Design review of the part built by this model. Coordinates are the model's own, in mm. Face numbers are marked on the shaded views. A direction names the side the tool comes from. Give positions to 0.01 mm unless a question says otherwise; leave off trailing zeros. Order: outer loops, then holes, each group sorted by start corner. A loop starts at its lowest first (then second) coordinate and runs counter-clockwise, first axis right, second up. Notation, with made-up numbers: (-26.5, 32) -> (10.5, 32) arc R28 ccw to (10.5, 66) -> close; hole circle Ø8 at (-15.75, -23). An arc over 180 degrees is marked (long way). Return JSON: item names as keys, results as strings.
```python
from build123d import *

# Parameters (mm, degrees)
BOSS_EXTRUDE1_DEPTH = 32
FILLET1_R           = 10
SKETCH4_W           = 170.11041037
SKETCH4_H           = 258.008077424
CUT_EXTRUDE2_DEPTH  = 33
SKETCH6_R           = 1.2
CUT_EXTRUDE3_DEPTH  = 61.218304139
SKETCH7_R           = 1.2
CUT_EXTRUDE4_DEPTH  = 61.218304139


with BuildPart() as part:
    # Sketch1 → Boss-Extrude1 (new body)
    with BuildSketch(Plane(origin=(0, 0, 0), x_dir=(1, 0, 0), z_dir=(0, 1, 0))):
        Polygon((0, 0), (0, 30), (83, 115), (83, 107.843231513), (5, 27.963713441), (5, -27.963713441), (83, -107.843231513), (83, -115), (0, -30), align=None)
    extrude(amount=BOSS_EXTRUDE1_DEPTH)

    # Fillet1
    fillet1_edges = [part.edges().sort_by_distance(p)[0] for p in [
        (0, 16, 30),
        (0, 16, -30),
    ]]
    fillet(fillet1_edges, radius=FILLET1_R)

    # Sketch4 → Cut-Extrude2 (cut, through all)
    with BuildSketch(Plane(origin=(0, 32, 0), x_dir=(1, 0, 0), z_dir=(0, 1, 0))):
        with Locations((35.635219957, -4.046970822)):
            Rectangle(SKETCH4_W, SKETCH4_H)
        Polygon((14.577370106, -37.771863549), (11, -41.265060241), (0, -41.265060241), (0, 41.265060241), (11, 41.265060241), (14.577370106, 37.771863549), align=None, mode=Mode.SUBTRACT)
    extrude(amount=-CUT_EXTRUDE2_DEPTH, mode=Mode.SUBTRACT)

    # Sketch6 → Cut-Extrude3 (cut, through all)
    with BuildSketch(Plane(origin=(-14.995748902, 0, -14.642907751), x_dir=(-0.698639338, 0, 0.715474021), z_dir=(-0.715474021, 0, -0.698639338))):
        with Locations((-34.209111306, 26)):
            Circle(SKETCH6_R)
        with Locations((-34.209111306, 6)):
            Circle(SKETCH6_R)
    extrude(amount=-CUT_EXTRUDE3_DEPTH, mode=Mode.SUBTRACT)

    # Sketch7 → Cut-Extrude4 (cut, through all)
    with BuildSketch(Plane(origin=(-14.995748902, 0, 14.642907751), x_dir=(0.698639338, 0, 0.715474021), z_dir=(-0.715474021, 0, 0.698639338))):
        with Locations((34.209111306, 26)):
            Circle(SKETCH7_R)
        with Locations((34.209111306, 6)):
            Circle(SKETCH7_R)
    extrude(amount=-CUT_EXTRUDE4_DEPTH, mode=Mode.SUBTRACT)


solid = part.part
```
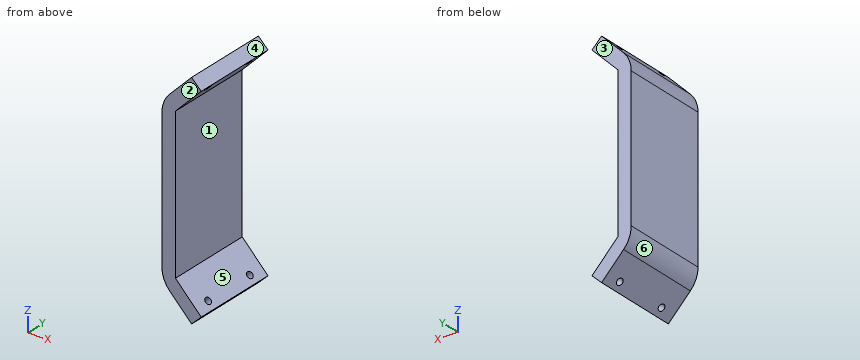
Item 1: Add section D-D (x = 1.25). Give the boundary of the cut face in (y, z), plus the area to 3 significant figures.
Result set:
{"outline": "(0, -30.77) -> (32, -30.77) -> (32, 30.77) -> (0, 30.77) -> close", "area": "1,970 mm^2"}
Item 2: For pin 1 (2 mm diameter, centred on x = 7.5, y = 28.5, fed in from +Z); pin 2 (4 mm diameter, centred on x = 4.5, y = 13, fed in from +Z); pin 3 (5 mm diameter, centred on y = 15, z = -1.5, fed in from +X), all flat-tipped, find the tip position at first contact; note any pin that passes through.
Result set:
{"pin 1": "stops at z = 38.7", "pin 2": "stops at z = 36.66", "pin 3": "stops at x = 5"}
Item 3: Add section C-C (z = 6). Give the boundary of the cut face in (x, y).
Result set:
{"outline": "(0, 0) -> (5, 0) -> (5, 32) -> (0, 32) -> close"}
Item 4: Add section A-A (x = 6). Give the boundary of the cut face in (y, z), plus the area to 3 significant figures.
Result set:
{"outline": "(0, -36.14) -> (32, -36.14) -> (32, -28.99) -> (0, -28.99) -> close; (0, 28.99) -> (32, 28.99) -> (32, 36.14) -> (0, 36.14) -> close", "area": "458 mm^2"}
Item 5: Mouldability with a two-part tool opening along Z and no side actions: class the marked faces 3, 4, 5 and 6 as released by +Z, released by -Z, zero draft, split by the parting line, or undercut.
Result set:
{"face 3": "zero draft", "face 4": "released by +Z", "face 5": "undercut", "face 6": "released by -Z"}
Item 6: Add section B-B (y = 16). Give the boundary of the cut face in (x, z), plus the area to 3 significant figures.
Result set:
{"outline": "(0, -25.93) arc R10 ccw to (2.85, -32.91) -> (11, -41.27) -> (14.58, -37.77) -> (5, -27.96) -> (5, 27.96) -> (14.58, 37.77) -> (11, 41.27) -> (2.85, 32.91) arc R10 ccw to (0, 25.93) -> close", "area": "433 mm^2"}
Item 7: Wall thickness on L1, parallel to X at y = 3, z = 24; L2, parallel to Z at x = 5.5, y = 22.5; L3, parallel to Z at x = 8.5, y = 22: over which ranges is each line inside the solid? List them lowest first. Write a range as [from, to].
Result set:
{"L1": "x = [0, 5]", "L2": "z = [-35.63, -28.48], [28.48, 35.63]", "L3": "z = [-38.7, -31.55], [31.55, 38.7]"}
Item 8: Machinability: for the marked faces 1 and 2, which of the approach directions +Z, -Z, +X, -X, +Y, -Y give a long, thin tool a straight path to every point of the face, cutting with its end or side? Answer none if there is none.
Result set:
{"face 1": "+X, +Y, -Y", "face 2": "+Z, -Z, +X, -X, -Y"}
